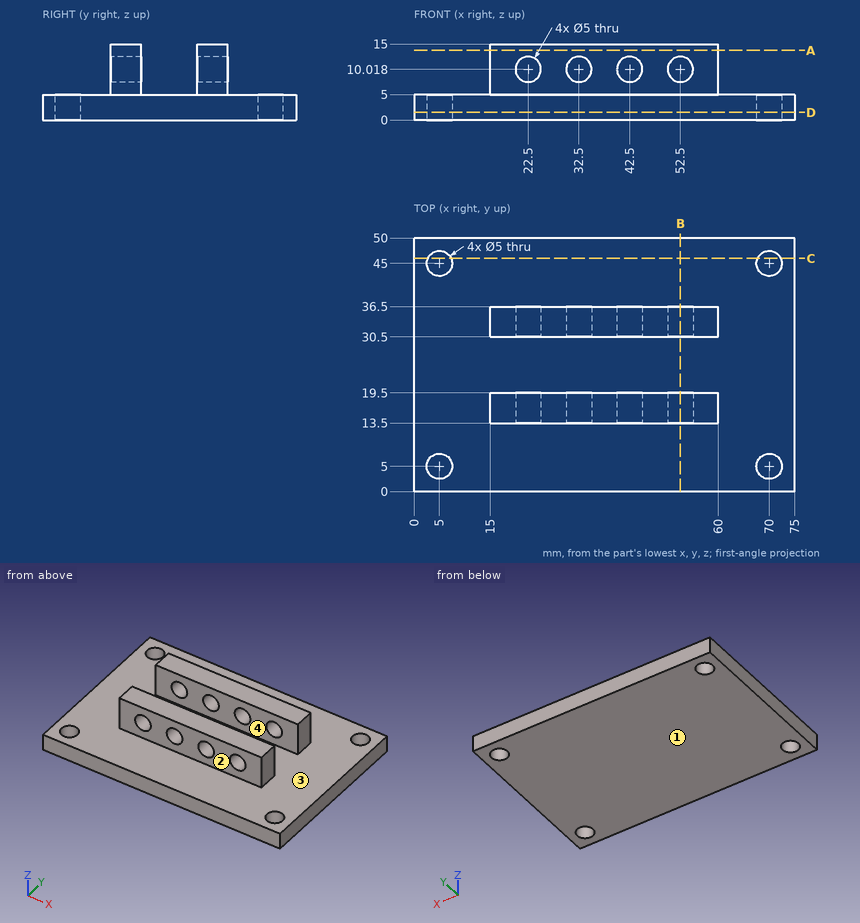
Verification items for this drawing (mm, ordinates from the low corner). Round coordinates to 2 decimals unless told otherwise and drop trailing zeros. Loops run counter-clockwise (first coordinate to the right, second up) from the corner with the lowest first, then second, coordinate; pieces in that order, holes last. Notation, with made-up numbers: (-15, -11) - (31, -11) arc R26 cw to (31, 3) - close; hole circle Ø4 at (74.25, 65.25). An arc over 180 degrees is marked (long way). Answer as CSV lines item,"result". Start each with the question number.
Item 1: Depth check by flat-ended pin: P1, Ø1.8, axis at y = 34.5, z = 9, coming from the +X side; P2, Ø1.5, axis at x = 30, z = 6.5, coming from the -Y side; P3, Ø3, axis at x = 39, z = 11.5, coming from the +Y side. Enter the tip coordinate at first touch or a pass-through.
Item 2: Scan lines: line 1 (Y direction, x = 70, z = 1.45); line 2 (Y direction, x = 37.5, z = 5.75); line 3 (Y direction, x = 4.5, z = 4). Record each from-to range of solid material in increasing order. Write a range as [from, to].
Item 3: Section check D-D (z = 1.5). Record the boundary of the cut face in (x, y).
Item 4: Section check B-B (x = 52.5). Record the boundary of the cut face in (y, z).
Item 5: Section check A-A (z = 13.75). Record the boundary of the cut face in (x, y), and give its area (3 significant figures).
Item 6: Section check C-C (y = 46). Record the boundary of the cut face in (x, z), and give its area (3 significant figures).
Item 7: Release check for a two-part mould opening along Y. For the marked faces 1, 2, 3 and 4 record: +Y half, -Y half, draft (parallel to the pull), parting line (faces both ways), or undercut.
Report:
1,P1,"stops at x = 60"
1,P2,"stops at y = 13.5"
1,P3,"stops at y = 36.5"
2,line 1,"y = [0, 2.5], [7.5, 42.5], [47.5, 50]"
2,line 2,"y = [13.5, 19.5], [30.5, 36.5]"
2,line 3,"y = [0, 2.55], [7.45, 42.55], [47.45, 50]"
3,outline,"(0, 0) - (75, 0) - (75, 50) - (0, 50) - close; hole circle Ø5 at (5, 5); hole circle Ø5 at (5, 45); hole circle Ø5 at (70, 5); hole circle Ø5 at (70, 45)"
4,outline,"(0, 0) - (50, 0) - (50, 5) - (36.5, 5) - (36.5, 7.52) - (30.5, 7.52) - (30.5, 5) - (19.5, 5) - (19.5, 7.52) - (13.5, 7.52) - (13.5, 5) - (0, 5) - close; (13.5, 12.52) - (19.5, 12.52) - (19.5, 15) - (13.5, 15) - close; (30.5, 12.52) - (36.5, 12.52) - (36.5, 15) - (30.5, 15) - close"
5,outline,"(15, 13.5) - (60, 13.5) - (60, 19.5) - (15, 19.5) - close; (15, 30.5) - (60, 30.5) - (60, 36.5) - (15, 36.5) - close"
5,area,"540 mm2"
6,outline,"(0, 0) - (2.71, 0) - (2.71, 5) - (0, 5) - close; (7.29, 0) - (67.71, 0) - (67.71, 5) - (7.29, 5) - close; (72.29, 0) - (75, 0) - (75, 5) - (72.29, 5) - close"
6,area,"329 mm2"
7,face 1,"draft"
7,face 2,"-Y half"
7,face 3,"undercut"
7,face 4,"undercut"
